from build123d import *

# Parameters (mm, degrees)
F0_W     = 110
F0_H     = 56
F0_W_2   = 80
F0_H_2   = 30
F1_DEPTH = 1.5
F2_R     = 3
F2_R_2   = 1
F3_DEPTH = 5


# Not quite as in the source:
# - a fillet or chamfer that OpenCascade refuses, or shapes differently, is made with other operations: its cross-section is extruded or revolved along the edge and cut away or added


with BuildPart() as f1:
    # F0 (on Top) → F1 (new body)
    with BuildSketch(Plane.XY):
        Rectangle(F0_W, F0_H)
        with Locations((0, 3)):
            Rectangle(F0_W_2, F0_H_2, mode=Mode.SUBTRACT)
    extrude(amount=F1_DEPTH)

    # F2 (on face) → F3 (join)
    with BuildSketch(Plane.XY.offset(1.5)):
        with Locations((-35.56, 24.13)):
            Circle(F2_R)
        with Locations((-35.56, 24.13)):
            Circle(F2_R_2, mode=Mode.SUBTRACT)
        with Locations((39.37, 24.13)):
            Circle(F2_R)
        with Locations((39.37, 24.13)):
            Circle(F2_R_2, mode=Mode.SUBTRACT)
        with Locations((-36.83, -24.13)):
            Circle(F2_R)
        with Locations((-36.83, -24.13)):
            Circle(F2_R_2, mode=Mode.SUBTRACT)
        with Locations((15.24, -19.05)):
            Circle(F2_R)
        with Locations((15.24, -19.05)):
            Circle(F2_R_2, mode=Mode.SUBTRACT)
        with Locations((45.72, -24.13)):
            Circle(F2_R)
        with Locations((45.72, -24.13)):
            Circle(F2_R_2, mode=Mode.SUBTRACT)
    extrude(amount=F3_DEPTH)

    # F4: chamfer of 1 on 10 edges, made by hand


with BuildPart() as f4_tool2:
    # F4_s3 → F4_t4 (revolve)
    with BuildSketch(Plane.XZ.offset(-24.13)):
        Polygon((-31.56, 1.5), (-32.56, 2.5), (-32.56, 1.5), align=None)
    revolve(axis=Axis((-35.56, 24.13, 1.5), (0, 0, 1)))

    split(bisect_by=Plane.XZ.offset(-28), keep=Keep.TOP)


with BuildPart() as f1_1:
    add(f1.part)

    # F4_t1: union F4_tool2
    add(f4_tool2.part)


with BuildPart() as f4_tool7:
    # F4_s8 → F4_t9 (revolve)
    with BuildSketch(Plane.XZ.offset(-24.13)):
        Polygon((43.37, 1.5), (42.37, 2.5), (42.37, 1.5), align=None)
    revolve(axis=Axis((39.37, 24.13, 1.5), (0, 0, 1)))

    split(bisect_by=Plane.XZ.offset(-28), keep=Keep.TOP)


with BuildPart() as f1_2:
    add(f1_1.part)

    # F4_t6: union F4_tool7
    add(f4_tool7.part)


with BuildPart() as f4_tool12:
    # F4_s13 → F4_t14 (revolve)
    with BuildSketch(Plane.XZ.offset(24.13)):
        Polygon((49.72, 1.5), (48.72, 2.5), (48.72, 1.5), align=None)
    revolve(axis=Axis((45.72, -24.13, 1.5), (0, 0, 1)))

    split(bisect_by=Plane.XZ.offset(28), keep=Keep.BOTTOM)


with BuildPart() as f1_3:
    add(f1_2.part)

    # F4_t11: union F4_tool12
    add(f4_tool12.part)

    # F4_s16 → F4_t17 (revolve)
    with BuildSketch(Plane.XZ.offset(19.05)):
        Polygon((19.24, 1.5), (18.24, 2.5), (18.24, 1.5), align=None)
    revolve(axis=Axis((15.24, -19.05, 1.5), (0, 0, 1)))


with BuildPart() as f4_tool19:
    # F4_s20 → F4_t21 (revolve)
    with BuildSketch(Plane.XZ.offset(24.13)):
        Polygon((-32.83, 1.5), (-33.83, 2.5), (-33.83, 1.5), align=None)
    revolve(axis=Axis((-36.83, -24.13, 1.5), (0, 0, 1)))

    split(bisect_by=Plane.XZ.offset(28), keep=Keep.BOTTOM)


with BuildPart() as f1_4:
    add(f1_3.part)

    # F4_t18: union F4_tool19
    add(f4_tool19.part)

    # F4_s23 → F4_t24 (revolve, cut)
    with BuildSketch(Plane.XZ.offset(24.13)):
        Polygon((-33.83, 5.5), (-34.83, 6.5), (-33.83, 6.5), align=None)
    revolve(axis=Axis((-36.83, -24.13, 6.5), (0, 0, 1)), mode=Mode.SUBTRACT)

    # F4_s25 → F4_t26 (revolve, cut)
    with BuildSketch(Plane.XZ.offset(-24.13)):
        Polygon((-32.56, 5.5), (-33.56, 6.5), (-32.56, 6.5), align=None)
    revolve(axis=Axis((-35.56, 24.13, 6.5), (0, 0, 1)), mode=Mode.SUBTRACT)

    # F4_s27 → F4_t28 (revolve, cut)
    with BuildSketch(Plane.XZ.offset(-24.13)):
        Polygon((42.37, 5.5), (41.37, 6.5), (42.37, 6.5), align=None)
    revolve(axis=Axis((39.37, 24.13, 6.5), (0, 0, 1)), mode=Mode.SUBTRACT)

    # F4_s29 → F4_t30 (revolve, cut)
    with BuildSketch(Plane.XZ.offset(24.13)):
        Polygon((48.72, 5.5), (47.72, 6.5), (48.72, 6.5), align=None)
    revolve(axis=Axis((45.72, -24.13, 6.5), (0, 0, 1)), mode=Mode.SUBTRACT)

    # F4_s31 → F4_t32 (revolve, cut)
    with BuildSketch(Plane.XZ.offset(19.05)):
        Polygon((18.24, 5.5), (17.24, 6.5), (18.24, 6.5), align=None)
    revolve(axis=Axis((15.24, -19.05, 6.5), (0, 0, 1)), mode=Mode.SUBTRACT)


solid = f1_4.part
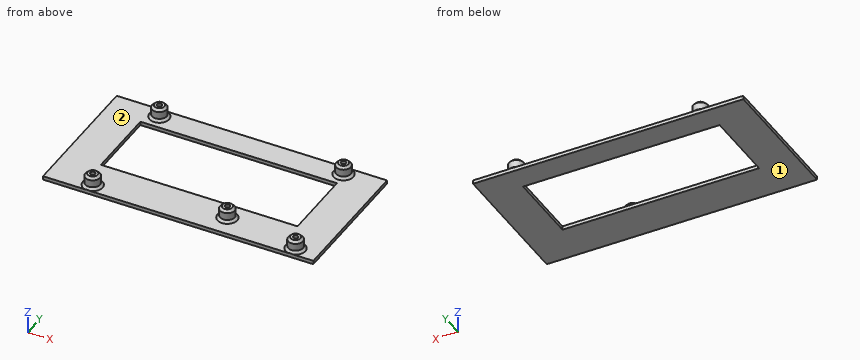
Check sheet for the modelled part. Datum: model origin and axes. Units: mm. Face numbers are marked on the shaded views. Round coordinates to 2 decimals unless told otherwise and drop trailing zeros. Loops run counter-clockwise (first coordinate to the right, second up) from the corner with the lowest first, then second, coordinate; pieces in that order, holes last.
1. Sectioned sample at C-C on x = 24. Record the boundary of the cut face in (y, z).
2. Sectioned sample at A-A on z = 4.5. Give the number of separate pieces and of enclosed holes in the cut face, and give its area (3 significant figures).
3. Sectioned sample at D-D on x = 45.72. Record the boundary of the cut face in (y, z), and give its area (3 significant figures).
4. Mould release check, pull along X, two halves, no side actions. Record for the marked faces 1 and 2: released by +X, released by -X, zero draft, split by the parting line, or undercut.
5. Sectioned sample at B-B on y = 7. Record the boundary of the cut face in (x, z), and give its area (3 significant figures).
6. Scan lines: probe 1 along Y at (x, z) = (-25.5, 0.5); probe 2 along Y at (x, z) = (45.72, 2.85); probe 3 along Y at (x, z) = (-35.56, 3.1). Record each from-to range of solid material in increasing order.
7. Gauge pin test, flat end, axial feed: pin 1 Ø0.6 at (x, y) = (-36, 24) entering from +Z. Record the tip position at first contact, or that the pin passes through.
Recorded:
1. outline: (-28, 0) - (-12, 0) - (-12, 1.5) - (-28, 1.5) - close; (18, 0) - (28, 0) - (28, 1.5) - (18, 1.5) - close
2. separate pieces: 5
2. enclosed holes: 5
2. area: 126 mm2
3. outline: (-28, 0) - (28, 0) - (28, 1.5) - (-20.13, 1.5) - (-21.13, 2.5) - (-21.13, 5.5) - (-22.13, 6.5) - (-23.13, 6.5) - (-23.13, 1.5) - (-25.13, 1.5) - (-25.13, 6.5) - (-26.13, 6.5) - (-27.13, 5.5) - (-27.13, 2.5) - (-28, 1.63) - close
3. area: 104 mm2
4. face 1: zero draft
4. face 2: undercut
5. outline: (-55, 0) - (-40, 0) - (-40, 1.5) - (-55, 1.5) - close; (40, 0) - (55, 0) - (55, 1.5) - (40, 1.5) - close
5. area: 45.0 mm2
6. probe 1: y = -28 to -12, 18 to 28
6. probe 2: y = -27.13 to -25.13, -23.13 to -21.13
6. probe 3: y = -26.85 to -21.41, 21.13 to 23.13, 25.13 to 27.13
7. pin 1: stops at z = 1.5
